from build123d import *

# Parameters (mm, degrees)
BOSS_EXTRUDE1_DEPTH                   = 1
BOSS_EXTRUDE1_DEPTH_BACK              = 19
SKETCH1_W                             = 50.25
SKETCH1_H                             = 30.25
BOSS_EXTRUDE2_DEPTH                   = 30.25
BOSS_EXTRUDE3_DEPTH                   = 5
M6_CLEARANCE_HOLE1_D                  = 6.6
M6_CLEARANCE_HOLE1_CSINK_D            = 6.65
M6_CLEARANCE_HOLE1_CSINK_ANGLE        = 90
SKETCH6_W                             = 4
SKETCH6_H                             = 4
BOSS_EXTRUDE4_DEPTH                   = 1
FILLET1_R                             = 10
TAP_DRILL_FOR_M4X0_7_TAP1_D           = 3.3
TAP_DRILL_FOR_M4X0_7_TAP1_CSINK_D     = 3.35
TAP_DRILL_FOR_M4X0_7_TAP1_CSINK_ANGLE = 90
CUT_EXTRUDE1_DEPTH                    = 92.330529534
CUT_EXTRUDE1_DEPTH_BACK               = 92.330529534
SKETCH13_OUTSIDE_W                    = 121.742
SKETCH13_OUTSIDE_H                    = 131.492
BOSS_EXTRUDE5_START                   = 21.26
BOSS_EXTRUDE5_DEPTH                   = 21.26
CUT_EXTRUDE2_DEPTH                    = 53.582495662
CUT_EXTRUDE2_DEPTH_BACK               = 53.582495662
SKETCH15_R                            = 1.65
BOSS_EXTRUDE6_REACH                   = 66.778
SKETCH16_W                            = 10
SKETCH16_H                            = 7
SKETCH17_W                            = 29.875
SKETCH17_H                            = 7
BOSS_EXTRUDE7_DEPTH                   = 20
FILLET5_R                             = 10
FILLET6_R                             = 3
SKETCH19_R                            = 2.75
CUT_EXTRUDE4_DEPTH                    = 64.502072703
FILLET7_R                             = 3
FILLET8_R                             = 10


with BuildPart() as part:
    # Sketch1 → Boss-Extrude1 (new, two sides: drawn at the far end of the back side and taken through both)
    with BuildSketch(Plane(origin=(0, 20.13, 0), x_dir=(1, 0, 0), z_dir=(0, 1, 0)).offset(-BOSS_EXTRUDE1_DEPTH_BACK)):
        Rectangle(SKETCH1_W, SKETCH1_H)
        Polygon((20.125, 10.125), (17.125, 10.125), (17.125, 11.125), (-17.125, 11.125), (-17.125, 10.125), (-20.125, 10.125), (-20.125, 7.125), (-21.125, 7.125), (-21.125, -7.125), (-20.125, -7.125), (-20.125, -10.125), (-17.125, -10.125), (-17.125, -11.125), (17.125, -11.125), (17.125, -10.125), (20.125, -10.125), (20.125, -7.125), (21.125, -7.125), (21.125, 7.125), (20.125, 7.125), align=None, mode=Mode.SUBTRACT)
    extrude(amount=BOSS_EXTRUDE1_DEPTH + BOSS_EXTRUDE1_DEPTH_BACK)

    # Sketch2 → Boss-Extrude2 (add)
    with BuildSketch(Plane.XY.offset(15.125)):
        Polygon((25.125, 21.13), (45.125, 21.13), (45.125, 61.13), (65.125, 61.13), (65.125, 1.13), (25.125, 1.13), align=None)
    extrude(amount=-BOSS_EXTRUDE2_DEPTH)

    # Sketch3 → Boss-Extrude3 (add)
    with BuildSketch(Plane(origin=(0, 61.13, 0), x_dir=(1, 0, 0), z_dir=(0, 1, 0))):
        with BuildLine():
            Line((65.125, 40), (65.125, -40))
            ThreePointArc((65.125, -40), (55.125, -50), (45.125, -40))
            Line((45.125, -40), (45.125, 40))
            ThreePointArc((45.125, 40), (55.125, 50), (65.125, 40))
        make_face()
    extrude(amount=-BOSS_EXTRUDE3_DEPTH)

    # M6 Clearance Hole1 (through all)
    with Locations(Plane(origin=(0, 56.13, 0), x_dir=(-1, 0, 0), z_dir=(0, -1, 0))):
        with Locations((-55.125, -40), (-55.125, 40)):
            CounterSinkHole(M6_CLEARANCE_HOLE1_D / 2, M6_CLEARANCE_HOLE1_CSINK_D / 2, counter_sink_angle=M6_CLEARANCE_HOLE1_CSINK_ANGLE)

    # Sketch6 → Boss-Extrude4 (add)
    with BuildSketch(Plane(origin=(0, 21.13, 0), x_dir=(1, 0, 0), z_dir=(0, 1, 0))):
        with Locations((19.125, 9.125)):
            Rectangle(SKETCH6_W, SKETCH6_H)
        with Locations((19.125, -9.125)):
            Rectangle(SKETCH6_W, SKETCH6_H)
        with Locations((-19.125, -9.125)):
            Rectangle(SKETCH6_W, SKETCH6_H)
        with Locations((-19.125, 9.125)):
            Rectangle(SKETCH6_W, SKETCH6_H)
    extrude(amount=-BOSS_EXTRUDE4_DEPTH)

    # Fillet1
    fillet1_edges = [part.edges().sort_by_distance(p)[0] for p in [
        (45.125, 21.13, 0),
        (65.125, 1.13, 0),
        (55.125, 56.13, -15.125),
        (55.125, 56.13, 15.125),
        (-25.125, 11.13, 15.125),
        (-25.125, 11.13, -15.125),
    ]]
    fillet(fillet1_edges, radius=FILLET1_R)

    # Tap Drill for M4x0.7 Tap1 (through all)
    with Locations(Plane(origin=(0, 1.13, 0), x_dir=(-1, 0, 0), z_dir=(0, -1, 0))):
        with Locations((-24.125, 0)):
            CounterSinkHole(TAP_DRILL_FOR_M4X0_7_TAP1_D / 2, TAP_DRILL_FOR_M4X0_7_TAP1_CSINK_D / 2, counter_sink_angle=TAP_DRILL_FOR_M4X0_7_TAP1_CSINK_ANGLE)

    # Sketch13 outside → Cut-Extrude1 (cut, two sides: drawn at the far end of the back side and taken through both)
    with BuildSketch(Plane(origin=(0, 21.13, 0), x_dir=(1, 0, 0), z_dir=(0, 1, 0)).offset(-CUT_EXTRUDE1_DEPTH_BACK)):
        with Locations((20, 0)):
            Rectangle(SKETCH13_OUTSIDE_W, SKETCH13_OUTSIDE_H)
        with BuildLine():
            Line((28.875, 5.125), (28.875, -5.125))
            ThreePointArc((28.875, -5.125), (25.946067812, -12.196067812), (18.875, -15.125))
            Line((18.875, -15.125), (-15.125, -15.125))
            ThreePointArc((-15.125, -15.125), (-22.196067812, -12.196067812), (-25.125, -5.125))
            Line((-25.125, -5.125), (-25.125, 5.125))
            ThreePointArc((-25.125, 5.125), (-22.196067812, 12.196067812), (-15.125, 15.125))
            Line((-15.125, 15.125), (18.875, 15.125))
            ThreePointArc((18.875, 15.125), (25.946067812, 12.196067812), (28.875, 5.125))
        make_face(mode=Mode.SUBTRACT)
    extrude(amount=CUT_EXTRUDE1_DEPTH + CUT_EXTRUDE1_DEPTH_BACK, mode=Mode.SUBTRACT)

    # Sketch14 → Boss-Extrude5 (add)
    with BuildSketch(Plane.XZ.offset(-1.13).offset(BOSS_EXTRUDE5_START)):
        with BuildLine():
            Line((28.875, 5.125), (28.875, -5.125))
            ThreePointArc((28.875, -5.125), (25.946067812, -12.196067812), (18.875, -15.125))
            Line((18.875, -15.125), (-15.125, -15.125))
            ThreePointArc((-15.125, -15.125), (-22.196067812, -12.196067812), (-25.125, -5.125))
            Line((-25.125, -5.125), (-25.125, 5.125))
            ThreePointArc((-25.125, 5.125), (-22.196067812, 12.196067812), (-15.125, 15.125))
            Line((-15.125, 15.125), (18.875, 15.125))
            ThreePointArc((18.875, 15.125), (25.946067812, 12.196067812), (28.875, 5.125))
        make_face()
        Polygon((-21.125, 7.125), (-20.125, 7.125), (-20.125, 10.125), (-17.125, 10.125), (-17.125, 11.125), (17.125, 11.125), (17.125, 10.125), (20.125, 10.125), (20.125, 7.125), (21.125, 7.125), (21.125, -7.125), (20.125, -7.125), (20.125, -10.125), (17.125, -10.125), (17.125, -11.125), (-17.125, -11.125), (-17.125, -10.125), (-20.125, -10.125), (-20.125, -7.125), (-21.125, -7.125), align=None, mode=Mode.SUBTRACT)
    extrude(amount=-BOSS_EXTRUDE5_DEPTH)

    # Sketch15 → Cut-Extrude2 (cut, two sides: drawn at the far end of the back side and taken through both)
    with BuildSketch(Plane(origin=(0, 21.13, 0), x_dir=(1, 0, 0), z_dir=(0, 1, 0)).offset(-CUT_EXTRUDE2_DEPTH_BACK)):
        with Locations(Location((24.125, 0, 0), (0, 0, 90))):
            Circle(SKETCH15_R)
    extrude(amount=CUT_EXTRUDE2_DEPTH + CUT_EXTRUDE2_DEPTH_BACK, mode=Mode.SUBTRACT)

    # Sketch16 → Boss-Extrude6 (add, up to next)
    with BuildSketch(Plane(origin=(28.875, 0, 13.75), x_dir=(0, 0, 1), z_dir=(-1, 0, 0)), mode=Mode.PRIVATE) as boss_extrude6_sk1:
        with Locations((-23.875, -16.63)):
            Rectangle(SKETCH16_W, SKETCH16_H)
    boss_extrude6_tool1 = extrude(boss_extrude6_sk1.sketch, amount=BOSS_EXTRUDE6_REACH, mode=Mode.PRIVATE) - part.part
    boss_extrude6 = boss_extrude6_tool1.solids().sort_by_distance((28.875, -16.63, -10.125))[0]
    add(boss_extrude6)

    # Sketch17 → Boss-Extrude7 (add)
    with BuildSketch(Plane.ZY.offset(-28.875)):
        with Locations((-30.0625, -16.63)):
            Rectangle(SKETCH17_W, SKETCH17_H)
    boss_extrude7 = extrude(amount=BOSS_EXTRUDE7_DEPTH)

    # Fillet5
    fillet5_edges = [part.edges().sort_by_distance(p)[0] for p in [
        (8.875, -16.63, -45),
        (28.875, -16.63, -45),
    ]]
    fillet(fillet5_edges, radius=FILLET5_R - 0.0001)  # a hair under: the kernel refuses the full size

    # Fillet6
    fillet6_edges = [part.edges().sort_by_distance(p)[0] for p in [
        (25.946067812, -13.13, -12.196067812),
        (13.875, -13.13, -15.125),
        (8.875, -16.63, -15.125),
    ]]
    fillet(fillet6_edges, radius=FILLET6_R)

    # Sketch19 → Cut-Extrude4 (cut, through all)
    with BuildSketch(Plane(origin=(0, -13.13, 0), x_dir=(1, 0, 0), z_dir=(0, 1, 0))):
        with Locations(Location((18.875, 35, 0), (0, 0, 270))):
            Circle(SKETCH19_R)
    cut_extrude4 = extrude(amount=-CUT_EXTRUDE4_DEPTH, mode=Mode.SUBTRACT)

    # Mirror2: Boss-Extrude6 across plane
    add(boss_extrude6.mirror(Plane.XY))

    # Mirror4: Boss-Extrude7 across plane
    add(boss_extrude7.mirror(Plane.XY))

    # Fillet7
    fillet7_edges = [part.edges().sort_by_distance(p)[0] for p in [
        (13.875, -13.13, 15.125),
        (25.946067812, -13.13, 12.196067812),
    ]]
    fillet(fillet7_edges, radius=FILLET7_R)
    fillet7_2_edges = [part.edges().sort_by_distance(p)[0] for p in [
        (8.875, -16.63, 15.125),
    ]]
    fillet(fillet7_2_edges, radius=FILLET7_R)

    # Fillet8
    fillet8_edges = [part.edges().sort_by_distance(p)[0] for p in [
        (8.875, -16.63, 45),
        (28.875, -16.63, 45),
    ]]
    fillet(fillet8_edges, radius=FILLET8_R - 0.0001)  # a hair under: the kernel refuses the full size

    # Mirror8: Cut-Extrude4 across plane
    add(cut_extrude4.mirror(Plane.XY), mode=Mode.SUBTRACT)


solid = part.part
Check sheet for the modelled part. Datum: model origin and axes. Units: mm. A direction names the side the tool comes from. Give positions to 0.01 mm unless a question says otherwise; leave off trailing zeros. Loops run counter-clockwise (first coordinate to the right, second up) from the corner with the lowest first, then second, coordinate; pieces in that order, holes last. Notation, with made-up numbers: M 57,2.25 L 100,2.25 A32 ccw 100,34.25 Z; hole C 49.25,-20 d3. An arc over 180 degrees is marked long. Answer as a JSON object with one key per item and string values. Group by question number.
Q1. Cross-section at A-A on y = 14. Give the number of separate pieces and of enclosed holes in the cut face, then the cut area to 3 significant figures.
Q2. Material ranges on line 1 along Z through (x, y) = (15, 11) (3 decimals); line 2 along X through (y, z) = (-16.5, -35) (3 decimals); line 3 along Y through (x, z) = (17.5, -18.5), recorded low to high. Write a range as [from, to].
Q3. Cross-section at C-C on z = -26.5. Record the cut outline in (x, y) (3 decimals).
Q4. Access from +Z, -Z, +X, -X, +Y, -Y to the whole of each face (thin tool, end or side, straight path). Record for faces 4 (the flat face through (8.875, -17, 27)), 5 (the flat face through (20.4, 1.9, 7.125)), 6 (the flat face through (-19, 20.13, -9)).
Q5. Go/stop test with flat-tipped pins: P1, Ø2, axis at y = -2.5, z = 14, coming from the +X side; P2, Ø3, axis at x = 18.5, y = 10.5, coming from the +Z side (3 decimals); P3, Ø1.5, axis at x = 18, z = -9, coming from the -Y side. Record where each tip stops, or that it passes through.
Q6. Release check for a two-part mould opening along X. For faces 1 (the flat face through (20.125, 0, -9)), 2 (the flat face through (2, 0, -15.125)), 3 (the cylindrical face through (8.02, -16.31, 16.03)) record: released by +X, released by -X, zero draft, split by the parting line, or undercut.
Q7. Cross-section at B-B on z = -3.5. Record the cut outline in (x, y) (3 decimals).
Evaluation:
{
 "1": {"separate pieces": "1", "enclosed holes": "2", "area": "627 mm2"},
 "2": {"line 1": "z = [-15.125, -11.125], [11.125, 15.125]", "line 2": "x = [8.875, 16.125], [21.625, 28.875]", "line 3": "y = [-20.13, -13.13]"},
 "3": {"outline": "M 8.875,-20.13 L 28.875,-20.13 L 28.875,-13.13 L 8.875,-13.13 Z"},
 "4": {"face 4": "+Z, -X, +Y, -Y", "face 5": "+Y, -Y", "face 6": "-Y"},
 "5": {"P1": "stops at x = 25.04", "P2": "stops at z = 15.125", "P3": "stops at y = 20.13"},
 "6": {"face 1": "undercut", "face 2": "zero draft", "face 3": "released by -X"},
 "7": {"outline": "M -25.125,-20.13 L -21.125,-20.13 L -21.125,21.13 L -25.125,21.13 Z; M 21.125,-20.13 L 28.875,-20.13 L 28.875,21.13 L 21.125,21.13 Z"}
}
